Work out the finished part from the listing and answer in its coordinate system (mm). A direction names the side the tool comes from. Round coordinates to 2 decimals unless told otherwise and drop trailing zeros. Order: outer loops, then holes, each group sorted by start corner. A loop starts at its lowest first (then second) coordinate and runs counter-clockwise, first axis right, second up. Notation, with made-up numbers: M 0.5,62 L 26.5,62 A25 ccw 26.5,76 Z; hole C 34.5,48.25 d4. An arc over 180 degrees is marked long. Return JSON: item names as keys, results as strings.
from build123d import *

# Parameters (mm, degrees)
SKETCH1_R                   = 1.5
Y_KSEKLIK_EKSTR_ZYON1_DEPTH = 2.5


with BuildPart() as part:
    # Sketch1 → Yükseklik-Ekstrüzyon1 (new, symmetric)
    with BuildSketch(Plane.XY):
        with BuildLine():
            Line((-43.160520199, 10.421906731), (-55.793069396, 10.421906731))
            ThreePointArc((-55.793069396, 10.421906731), (-59.061190769, 12.033165476), (-59.773103822, 15.606672417))
            ThreePointArc((-59.773103822, 15.606672417), (-110.527372239, 79.765345936), (-157.455994445, 12.757618261))
            ThreePointArc((-157.455994445, 12.757618261), (-158.027333354, 9.050297499), (-161.3672053, 7.34269369))
            Line((-161.3672053, 7.34269369), (-174.920520263, 7.34269369))
            ThreePointArc((-174.920520263, 7.34269369), (-177.833800201, 8.549413752), (-179.040520263, 11.46269369))
            Line((-179.040520263, 11.46269369), (-179.040520263, 28.787024355))
            ThreePointArc((-179.040520263, 28.787024355), (-109.040520263, 98.787024355), (-39.040520263, 28.787024355))
            Line((-39.040520263, 28.787024355), (-39.040520263, 14.54118218))
            ThreePointArc((-39.040520263, 14.54118218), (-40.247496439, 11.628370637), (-43.160520199, 10.421906731))
        make_face()
        with Locations((-169.040520263, 15.783267045)):
            Circle(SKETCH1_R, mode=Mode.SUBTRACT)
        with Locations((-49.040520263, 15.783267045)):
            Circle(SKETCH1_R, mode=Mode.SUBTRACT)
        with Locations((-109.040520263, 89.703931552)):
            Circle(SKETCH1_R, mode=Mode.SUBTRACT)
    extrude(amount=Y_KSEKLIK_EKSTR_ZYON1_DEPTH, both=True)


solid = part.part
Item 1: Find section D-D (x = -90). Determine the outline of the cut face in (y, z), plus the area to 3 significant figures.
Output:
{"outline": "M 76.1,-2.5 L 96.15,-2.5 L 96.15,2.5 L 76.1,2.5 Z", "area": "100 mm^2"}
Item 2: Consider line 1 along X through (y, z) = (28.5, 1); line 2 along X through (y, z) = (45.5, 1.75); line 3 along Y through (x, z) = (-108.5, 2.05). Determine where each line is inside the solid, lowest interval first. Write a range as [from, to].
Output:
{"line 1": "x = [-179.04, -160.04], [-58.04, -39.04]", "line 2": "x = [-177.02, -157.22], [-60.86, -41.06]", "line 3": "y = [79.78, 88.3], [91.1, 98.78]"}
Item 3: Which of the six approach directions +Z, -Z, +X, -X, +Y, -Y give full straight-line access (tool end or side, diameter ignored) to faces 5 (the flat face through (-179.041, 20, 0)), 6 (the cylindrical face through (-158, 9.09, 0.04)), 7 (the flat face through (-49, 10.422, 0))?
Output:
{"face 5": "+Z, -Z, -X, +Y, -Y", "face 6": "+Z, -Z", "face 7": "+Z, -Z, +X, -Y"}
Item 4: Find section A-A (y = 31.5). Determine the outline of the cut face in (x, z).
Output:
{"outline": "M -178.99,-2.5 L -159.97,-2.5 L -159.97,2.5 L -178.99,2.5 Z; M -58.11,-2.5 L -39.09,-2.5 L -39.09,2.5 L -58.11,2.5 Z"}
Item 5: Each of these flat-tipped pins is pushed along its axis until it touches: pin 1 (1.5 mm diameter, centred on x = -125.5, z = -1, fed in from -Y); pin 2 (2.5 mm diameter, centred on x = -48.5, z = -0.5, fed in from -Y); pin 3 (2 mm diameter, centred on x = -157.5, y = 22.5, fed in from -Z). Where does it stop, or does it pass through?
Output:
{"pin 1": "stops at y = 76.8", "pin 2": "stops at y = 10.42", "pin 3": "passes through"}
Item 6: The mould has two halves that part along X. Classify faces 1 (the cylindrical face through (-170.54, 15.85, -0.04)), 2 (the cylindrical face through (-110.58, 98.77, 0.04)), 3 (the cylindrical face through (-40.216, 11.661, 0.035)), 4 (the flat face through (-168, 7.343, 0)): pulls with the +X half, pulls with the -X half, needs draft (parallel to the pull), parting line crosses it, or undercut.
Output:
{"face 1": "undercut", "face 2": "parting line crosses it", "face 3": "pulls with the +X half", "face 4": "needs draft"}
Item 7: Find section C-C (z = 0.9). Determine the outline of the cut face in (x, y).
Output:
{"outline": "M -179.04,11.46 A4.12 ccw -174.92,7.34 L -161.37,7.34 A4.12 ccw -157.46,12.76 A51 cw long -59.77,15.61 A4.12 ccw -55.79,10.42 L -43.16,10.42 A4.12 ccw -39.04,14.54 L -39.04,28.79 A70 ccw -179.04,28.79 Z; hole C -169.04,15.78 d3; hole C -109.04,89.7 d3; hole C -49.04,15.78 d3"}
Item 8: Find section B-B (x = -169). Determine the outline of the cut face in (y, z).
Output:
{"outline": "M 7.34,-2.5 L 14.28,-2.5 L 14.28,2.5 L 7.34,2.5 Z; M 17.28,-2.5 L 64.91,-2.5 L 64.91,2.5 L 17.28,2.5 Z"}
